Design review of the part shown in the three views and the two pictorial views. Dimensions are in mm from the part's minimum x, y and z. A direction names the side the tool comes from. Give positions to 0.01 mm unless a question says otherwise; leave off trailing zeros. Order: outer loops, then holes, each group sorted by start corner. A loop starts at its lowest first (then second) coordinate and runs counter-clockwise, first axis right, second up. Notation, with made-up numbers: (-34.75, -6.75) -> (-0.75, -6.75) arc R23 ccw to (-0.75, 26.25) -> close; hole circle Ø4 at (-17.75, -7). An arc over 180 degrees is marked (long way). Use one line per item in the form item = value.
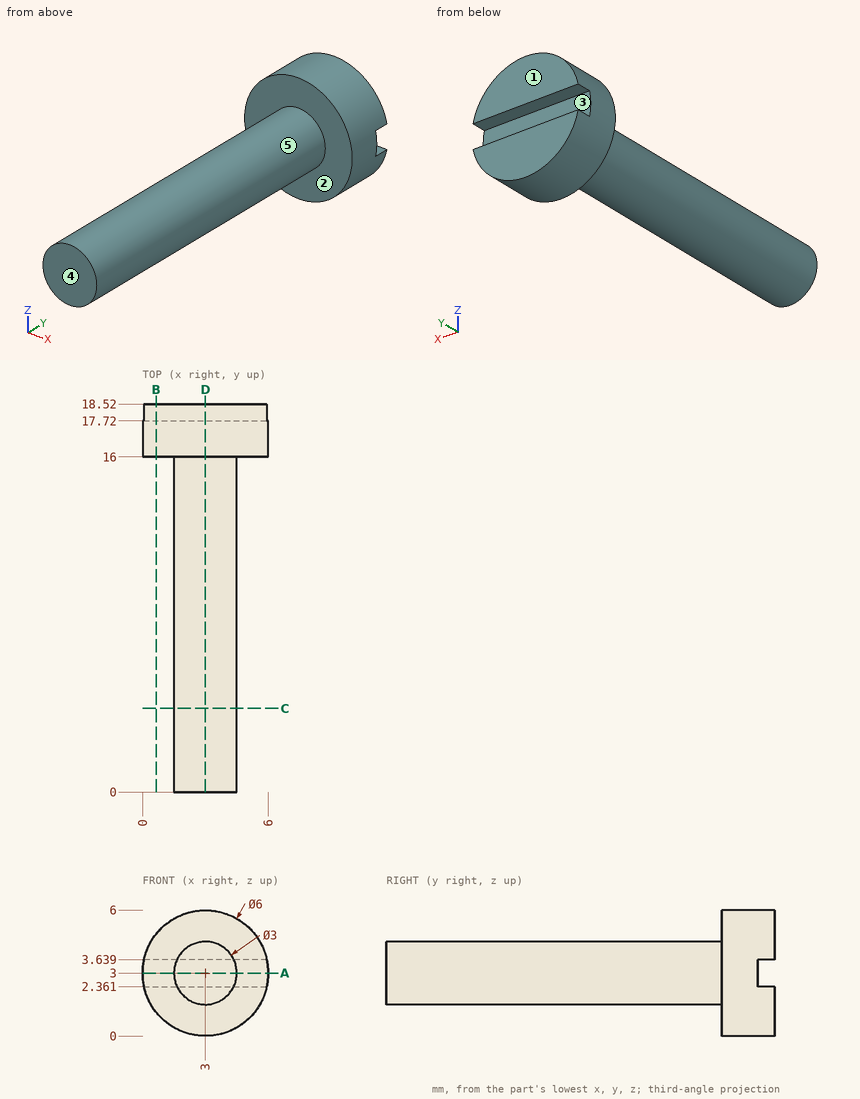
1. Add section B-B on x = 0.65. Give the boundary of the cut face in (y, z) (1 decimal).
Values:
outline = (16, 1.1) -> (18.5, 1.1) -> (18.5, 2.4) -> (17.7, 2.4) -> (17.7, 3.6) -> (18.5, 3.6) -> (18.5, 4.9) -> (16, 4.9) -> close
2. Add section A-A on z = 3. Give the boundary of the cut face in (x, y).
Values:
outline = (0, 16) -> (1.5, 16) -> (1.5, 0) -> (4.5, 0) -> (4.5, 16) -> (6, 16) -> (6, 17.72) -> (0, 17.72) -> close
3. Add section C-C on y = 4. Give the boundary of the cut face in (x, z).
Values:
outline = circle Ø3 at (3, 3)
4. Tool access review of the marked faces 1 and 2: name each direction out of +Z, -Z, +X, -X, +Y, -Y from which nothing blocks a thin tool from reaching the whole face with its end or side.
Values:
face_1 = +Z, -Z, +X, -X, +Y
face_2 = -Y
5. Add section D-D on x = 3. Give the boundary of the cut face in (y, z), then the cut area to 3 significant figures.
Values:
outline = (0, 1.5) -> (16, 1.5) -> (16, 0) -> (18.52, 0) -> (18.52, 2.36) -> (17.72, 2.36) -> (17.72, 3.64) -> (18.52, 3.64) -> (18.52, 6) -> (16, 6) -> (16, 4.5) -> (0, 4.5) -> close
area = 62.1 mm^2
6. The part is to be moulded in two halves that separate along Z. For the marked faces 3, 4 and 5, say which applies: +Z half, -Z half, draft (parallel to the pull), parting line (faces both ways), or undercut.
Values:
face_3 = undercut
face_4 = draft
face_5 = parting line
7. For pin 1 Ø1.5 at (y, z) = (10.5, 3) entering from +X; pin 2 Ø3 at (x, y) = (3, 10) entering from +Z; pin 3 Ø3 at (x, z) = (3, 1) entering from -Y; pin 4 Ø0.6 at (x, z) = (4, 3) entering from +Y, all flat-tipped, find the tip position at first contact; note any pin that passes through.
Values:
pin_1 = 4.5
pin_2 = 4.5
pin_3 = 0
pin_4 = 17.72
8. For L1, parallel to Y at x = 4.4, z = 4.55; L2, parallel to Y at x = 4.2, z = 2.4; L3, parallel to X at y = 9, z = 4.25, list the stretches that pass through material, from the lowest coordinate up.
Values:
L1 = 16 to 18.52
L2 = 0 to 17.72
L3 = 2.17 to 3.83
